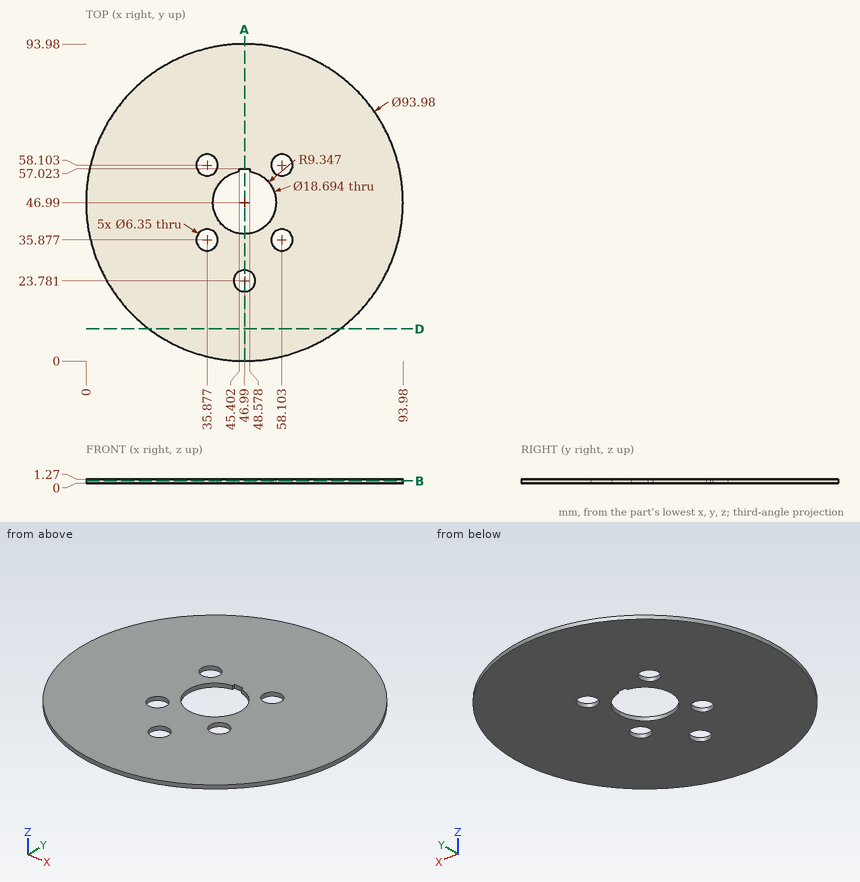
Can you work these out from the drawing? Everything is in mm from the part's minimum corner. Give positions to 0.01 mm unless a question says otherwise; leave off trailing zeros. Loops run counter-clockwise (first coordinate to the right, second up) from the corner with the lowest first, then second, coordinate; pieces in that order, holes last. Notation, with made-up numbers: (76.25, -23) - (110.25, -23) arc R15 cw to (110.25, -15) - close; hole circle Ø8 at (34, 53). An arc over 180 degrees is marked (long way). Answer as a JSON object with one key per item and string values.
Q1. Imagine slicing it at B-B on z = 0.7. Give the number of separate pieces and of enclosed holes in the cut face, plus the area to 3 significant figures.
Geometry says:
{"separate pieces": "1", "enclosed holes": "6", "area": "6,500 mm²"}
Q2. If I drill on L1, parallel to Y at x = 46.99, z = 0.95 (1 decimal); L2, parallel to X at y = 47, z = 0.9; L3, parallel to Y at x = 48, z = 0.15, over which ranges is the centre line in solid material (lowest first)?
Geometry says:
{"L1": "0 to 20.6, 27 to 37.6, 57 to 94", "L2": "0 to 37.64, 56.34 to 93.98", "L3": "0.01 to 20.77, 26.79 to 37.7, 57.02 to 93.97"}
Q3. Imagine slicing it at D-D on y = 9.5. Write out the boundary of the cut face in (x, z).
Geometry says:
{"outline": "(18.66, 0) - (75.32, 0) - (75.32, 1.27) - (18.66, 1.27) - close"}
Q4. Imagine slicing it at A-A on x = 46.99. Write out the boundary of the cut face in (y, z) (1 decimal).
Geometry says:
{"outline": "(0, 0) - (20.6, 0) - (20.6, 1.3) - (0, 1.3) - close; (27, 0) - (37.6, 0) - (37.6, 1.3) - (27, 1.3) - close; (57, 0) - (94, 0) - (94, 1.3) - (57, 1.3) - close"}
Q5. Will these pins go through, and if not, where does the flat tip stop? P1, Ø6, axis at x = 36, y = 73, coming from the -Z side; P2, Ø0.6, axis at x = 47.5, z = 1, coming from the -Y side.
Geometry says:
{"P1": "z = 0", "P2": "y = 0"}
